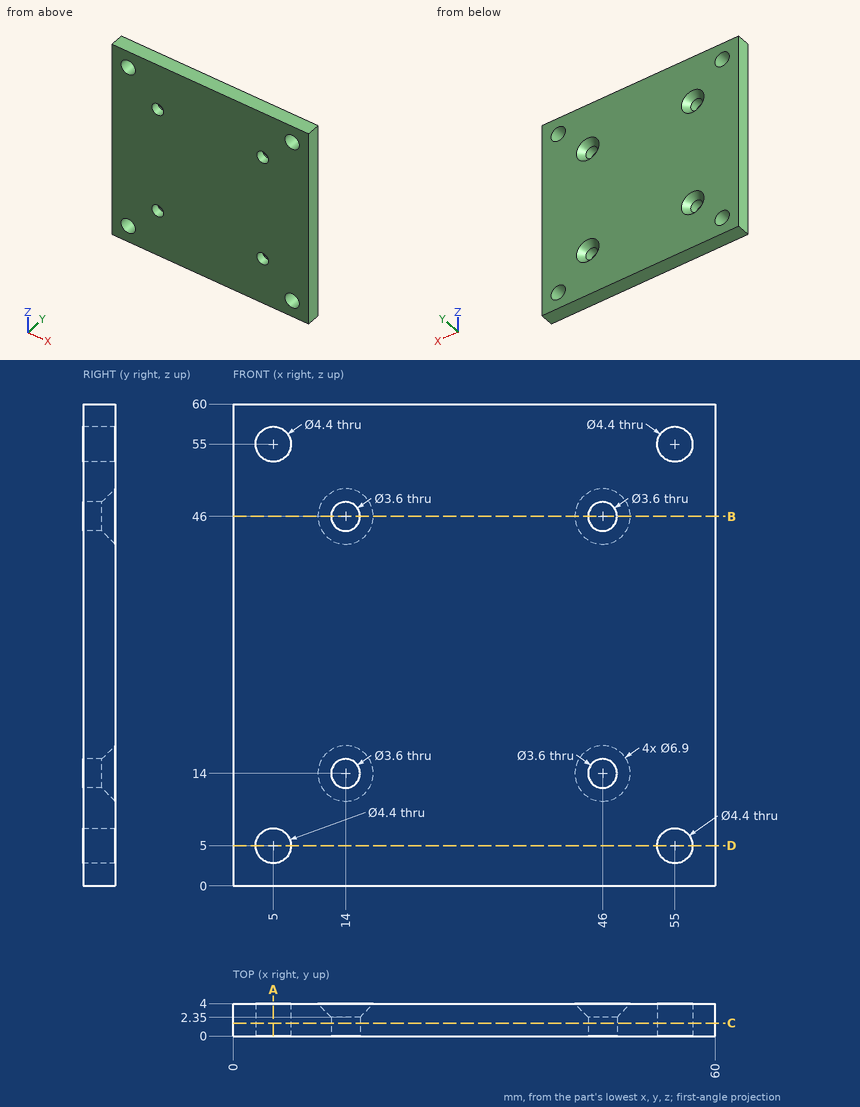
Drawing for the job (mm, zero at the part's lowest x, y, z). Give positions to 0.01 mm unless a question says otherwise; leave off trailing zeros. Loops run counter-clockwise (first coordinate to the right, second up) from the corner with the lowest first, then second, coordinate; pieces in that order, holes last.
(1) Drill centre lines: line 1 along X through (y, z) = (1.95, 46); line 2 along X through (y, z) = (1.8, 5). Where is each one in solid material? Low to high.
Return value:
line 1: x = 0 to 12.2, 15.8 to 44.2, 47.8 to 60
line 2: x = 0 to 2.8, 7.2 to 52.8, 57.2 to 60
(2) Band-saw the part on D-D (z = 5). Write the cut outline in (x, y), and give its area (3 significant figures).
Return value:
outline: (0, 0) - (2.8, 0) - (2.8, 4) - (0, 4) - close; (7.2, 0) - (52.8, 0) - (52.8, 4) - (7.2, 4) - close; (57.2, 0) - (60, 0) - (60, 4) - (57.2, 4) - close
area: 205 mm2
(3) Band-saw the part on B-B (z = 46). Write the cut outline in (x, y).
Return value:
outline: (0, 0) - (12.2, 0) - (12.2, 2.35) - (10.55, 4) - (0, 4) - close; (15.8, 0) - (44.2, 0) - (44.2, 2.35) - (42.55, 4) - (17.45, 4) - (15.8, 2.35) - close; (47.8, 0) - (60, 0) - (60, 4) - (49.45, 4) - (47.8, 2.35) - close
(4) Band-saw the part on C-C (y = 1.6). Count the separate pieces of the cut face and the enclosed holes in it, and give its area (3 significant figures).
Return value:
separate pieces: 1
enclosed holes: 8
area: 3,500 mm2
(5) Pin check, flat tip, straight feed: pin 1 (4.5 mm diameter, centred on x = 46, z = 46, fed in from +Y). Stop position of the tip, or through.
Return value:
pin 1: stops at y = 2.8
(6) Band-saw the part on A-A (x = 5). Write the cut outline in (y, z), and give its area (3 significant figures).
Return value:
outline: (0, 0) - (4, 0) - (4, 2.8) - (0, 2.8) - close; (0, 7.2) - (4, 7.2) - (4, 52.8) - (0, 52.8) - close; (0, 57.2) - (4, 57.2) - (4, 60) - (0, 60) - close
area: 205 mm2
